CAD build for the part. Positions are in the model's coordinates, mm. A direction names the side the tool comes from. Coordinates: 2 decimals unless noted, no trailing zeros. Order: outer loops, then holes, each group sorted by start corner. A loop starts at its lowest first (then second) coordinate and runs counter-clockwise, first axis right, second up. Notation, with made-up numbers: (32, 45) - (66, 45) arc R11 ccw to (66, 56) - close; hole circle Ø3 at (-11.75, -21.5). An arc over 180 degrees is marked (long way). Use one line per item in the form item = value.
```python
from build123d import *

# Parameters (mm, degrees)
SWEEP1_PROFILE_R     = 13.49375
CUT_SWEEP1_PROFILE_R = 9.525


with BuildPart() as part:
    # Sweep1: sweep along a curve in space
    with BuildLine() as sweep1_path:
        Line((0, 0, 0), (0, 50.8, 0))
        ThreePointArc((0, 50.8, 0), (2.900189811, 65.380238773, 0), (11.159231637, 77.740768363, 0))
        Line((11.159231637, 77.740768363, 0), (25.4, 91.981536726, 0))
    # Sweep1 profile (on start of the path) → Sweep1 (sweep)
    with BuildSketch(Plane.ZX):
        Circle(SWEEP1_PROFILE_R)
    sweep(path=sweep1_path.line)

    # Cut-Sweep1: sweep along a curve in space
    with BuildLine() as cut_sweep1_path:
        Line((0, 0, 0), (0, 50.8, 0))
        ThreePointArc((0, 50.8, 0), (2.900189811, 65.380238773, 0), (11.159231637, 77.740768363, 0))
        Line((11.159231637, 77.740768363, 0), (25.4, 91.981536726, 0))
    # Cut-Sweep1 profile (on start of the path) → Cut-Sweep1 (sweep, cut)
    with BuildSketch(Plane.ZX):
        Circle(CUT_SWEEP1_PROFILE_R)
    sweep(path=cut_sweep1_path.line, mode=Mode.SUBTRACT)


solid = part.part
```
Item 1: Drop flat-ended pins along their axis: pin 1 (1.5 mm diameter, centred on y = 72.5, z = 4, fed in from +X); pin 2 (12 mm diameter, centred on y = 23, z = -7.5, fed in from +X); pin 3 (12 mm diameter, centred on y = 42.5, z = 0.5, fed in from -X); pin 4 (6 mm diameter, centred on x = 25.5, z = -1, fed in from +Y). Give the stop position or say it passes through.
Derived:
pin_1 = 24.96
pin_2 = 13.41
pin_3 = -13.49
pin_4 = 81.75
Item 2: 3-axis set-ups, long thin cutter, end or side, ignore diameter. For faces 1 (the face through (-5.796, 25.756, -7.559)), 2 (the face through (9.914, 93.426, 6.227)): which of +Z, -Z, +X, -X, +Y, -Y reach the whole face in a straight line?
Derived:
face_1 = -Y
face_2 = none
Item 3: Drill centre lines: line 1 (X direction, y = 38, z = 0) (3 decimals); line 2 (X direction, y = 60, z = 4.75); line 3 (Z direction, x = 3.5, y = 7). Where is each one in solid material? Low to high. Write a range as [from, to].
Derived:
line_1 = [-13.494, -9.525], [9.525, 13.494]
line_2 = [-11.79, -7.33], [9.71, 14.35]
line_3 = [-13.03, -8.86], [8.86, 13.03]
Item 4: Two-plate mould, pull along X, no slides. Class faces 3 (the face through (24.06, 79.28, 5.12)), 4 (the face through (9.12, 25.756, -9.945)), 5 (the face through (9.2, 0, -3.2)): +X half, -X half, draft (parallel to the pull), parting line (faces both ways), or undercut.
Derived:
face_3 = undercut
face_4 = parting line
face_5 = draft
Item 5: Cut at A-A, the plane z = -6.25. Write the cut outline in (x, y), plus the area to 3 significant figures.
Derived:
outline = (-11.96, 0) - (-7.19, 0) - (-7.19, 50.8) arc R45.29 cw to (6.08, 82.82) - (20.32, 97.06) - (16.94, 100.44) - (2.7, 86.2) arc R50.06 ccw to (-11.96, 50.8) - close; (7.19, 0) - (11.96, 0) - (11.96, 50.8) arc R26.14 cw to (19.62, 69.28) - (33.86, 83.53) - (30.48, 86.9) - (16.24, 72.66) arc R30.91 ccw to (7.19, 50.8) - close
area = 963 mm²
Item 6: Cut at D-D, the plane z = 10.75. Write the cut outline in (x, y).
Derived:
outline = (-8.16, 0) - (8.16, 0) - (8.16, 50.8) arc R29.94 cw to (16.93, 71.97) - (31.17, 86.21) - (19.63, 97.75) - (5.39, 83.51) arc R46.26 ccw to (-8.16, 50.8) - close
Item 7: Cut at C-C, the plane z = 1.25. Write the cut outline in (x, y), plus the area to 3 significant figures.
Derived:
outline = (-13.44, 0) - (-9.44, 0) - (-9.44, 50.8) arc R47.54 cw to (4.48, 84.42) - (18.72, 98.66) - (15.9, 101.48) - (1.66, 87.24) arc R51.54 ccw to (-13.44, 50.8) - close; (9.44, 0) - (13.44, 0) - (13.44, 50.8) arc R24.66 cw to (20.66, 68.24) - (34.9, 82.48) - (32.08, 85.3) - (17.84, 71.06) arc R28.66 ccw to (9.44, 50.8) - close
area = 806 mm²
